Part print with two shaded views. Sizes in mm from the minimum x, y, z corner. Give positions to 0.01 mm unless a question says otherwise; leave off trailing zeros. Write each loop counter-clockwise with the first axis right and the second up, starting at its lowest first coordinate (ties: lowest second). Pieces come first, ordered by that corner, then holes.
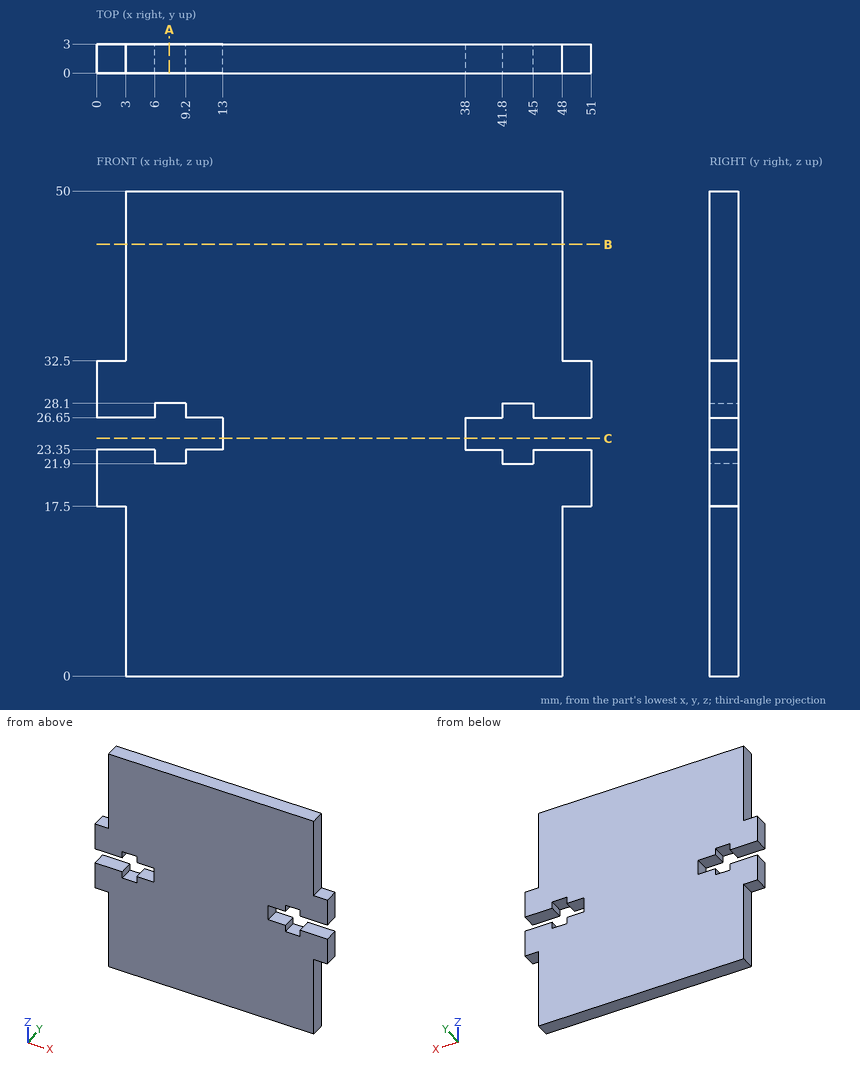
(1) Saw through at B-B, the plane z = 44.5. List the corners of the cut face in (x, y), plus the area to 3 significant figures.
(2) Saw through at A-A, the plane x = 7.5. List the corners of the cut face in (y, z).
(3) Saw through at C-C, the plane z = 24.5. List the corners of the cut face in (x, y).
(4) Probe line 1 (Z direction, x = 40.5, y = 2.65); line 2 (Z direction, x = 49, y = 2.1); line 3 (X direction, y = 1.3, z = 3). List the from-to ranges inside material, lowest first.
(5) Drop flat-ended pins along their axis: pin 1 (6 mm diameter, centred on x = 28, z = 22, fed in from -Y); pin 2 (1.5 mm diameter, centred on y = 1, z = 42.5, fed in from -X); pin 3 (1.5 mm diameter, centred on x = 1, y = 2, fed in from -Z); pin 4 (1.5 mm diameter, centred on x = 50, y = 2, fed in from +Z). Give the stop position or say it passes through.
Computed values:
1. outline: (3, 0) - (48, 0) - (48, 3) - (3, 3) - close
1. area: 135 mm2
2. outline: (0, 0) - (3, 0) - (3, 21.9) - (0, 21.9) - close; (0, 28.1) - (3, 28.1) - (3, 50) - (0, 50) - close
3. outline: (13, 0) - (38, 0) - (38, 3) - (13, 3) - close
4. line 1: z = 0 to 23.35, 26.65 to 50
4. line 2: z = 17.5 to 23.35, 26.65 to 32.5
4. line 3: x = 3 to 48
5. pin 1: stops at y = 0
5. pin 2: stops at x = 3
5. pin 3: stops at z = 17.5
5. pin 4: stops at z = 32.5
